The listing builds one solid part. Answer for the finished solid, in the listing's coordinates (mm). A direction names the side the tool comes from. Give positions to 0.01 mm unless a question says otherwise; leave off trailing zeros. Order: outer loops, then holes, each group sorted by start corner. A loop starts at its lowest first (then second) coordinate and runs counter-clockwise, first axis right, second up.
```python
from build123d import *

# Parameters (mm, degrees)
F1_DEPTH = 12.7
F3_DEPTH = 25.4
F4_R     = 4.8895
F5_DEPTH = 25.4


with BuildPart() as f1:
    # F0 (on Top) → F1 (new body)
    with BuildSketch(Plane.XY):
        Polygon((222.6329271213, 5.3004485337), (222.6329271213, 0), (222.6329271213, -5.3004485337), (222.6329271213, -30.3229389596), (285.3670728787, -30.3229389596), (285.3670728787, 30.3229389596), (222.6329271213, 30.3229389596), align=None)
        with BuildLine():
            ThreePointArc((44.1328420266, 5.3004485337), (44.3706396623, 2.654964399), (44.45, 0))
            Line((44.45, 0), (222.6329271213, 0))
            Line((222.6329271213, 0), (222.6329271213, 5.3004485337))
            Line((222.6329271213, 5.3004485337), (44.1328420266, 5.3004485337))
        make_face()
        with BuildLine():
            Line((222.6329271213, 0), (44.45, 0))
            ThreePointArc((44.45, 0), (44.3706396623, -2.654964399), (44.1328420266, -5.3004485337))
            Line((44.1328420266, -5.3004485337), (222.6329271213, -5.3004485337))
            Line((222.6329271213, -5.3004485337), (222.6329271213, 0))
        make_face()
        with BuildLine():
            ThreePointArc((-38.8833935549, 5.3004485337), (0, 39.243), (38.8833935548, 5.3004485337))
            Line((38.8833935548, 5.3004485337), (44.1328420266, 5.3004485337))
            ThreePointArc((44.1328420266, 5.3004485337), (0, 44.45), (-44.1328420266, 5.3004485337))
            Line((-44.1328420266, 5.3004485337), (-38.8833935549, 5.3004485337))
        make_face()
        with BuildLine():
            Line((44.1328420266, -5.3004485337), (38.8833935548, -5.3004485337))
            ThreePointArc((38.8833935548, -5.3004485337), (0, -39.243), (-38.8833935549, -5.3004485337))
            Line((-38.8833935549, -5.3004485337), (-44.1328420266, -5.3004485337))
            ThreePointArc((-44.1328420266, -5.3004485337), (0, -44.45), (44.1328420266, -5.3004485337))
        make_face()
        with BuildLine():
            ThreePointArc((38.8833935548, 5.3004485337), (39.1529951745, 2.656316597), (39.243, 0))
            Line((39.243, 0), (44.45, 0))
            ThreePointArc((44.45, 0), (44.3706396623, 2.654964399), (44.1328420266, 5.3004485337))
            Line((44.1328420266, 5.3004485337), (38.8833935548, 5.3004485337))
        make_face()
        with BuildLine():
            Line((44.45, 0), (39.243, 0))
            ThreePointArc((39.243, 0), (39.1529951745, -2.656316597), (38.8833935548, -5.3004485337))
            Line((38.8833935548, -5.3004485337), (44.1328420266, -5.3004485337))
            ThreePointArc((44.1328420266, -5.3004485337), (44.3706396623, -2.654964399), (44.45, 0))
        make_face()
        with BuildLine():
            ThreePointArc((-38.8833935549, -5.3004485337), (-39.243, 0), (-38.8833935549, 5.3004485337))
            Line((-38.8833935549, 5.3004485337), (-44.1328420266, 5.3004485337))
            ThreePointArc((-44.1328420266, 5.3004485337), (-44.45, 0), (-44.1328420266, -5.3004485337))
            Line((-44.1328420266, -5.3004485337), (-38.8833935549, -5.3004485337))
        make_face()
    extrude(amount=F1_DEPTH)

    # F2 (on face) → F3 (cut)
    with BuildSketch(Plane.XY.offset(12.7)):
        with BuildLine():
            ThreePointArc((261.2282336072, -15.141530461), (269.1570726001, -9.3443922439), (272.182900235, 0))
            ThreePointArc((272.182900235, 0), (269.1570726001, 9.3443922439), (261.2282336072, 15.141530461))
            Line((261.2282336072, 15.141530461), (261.2282336072, -15.141530461))
        make_face()
    extrude(amount=-F3_DEPTH, mode=Mode.SUBTRACT)

    # F4 (on face) → F5 (cut)
    with BuildSketch(Plane.YZ.offset(285.3670728787)):
        with Locations((0, 6.35)):
            Circle(F4_R)
    extrude(amount=-F5_DEPTH, mode=Mode.SUBTRACT)


solid = f1.part
```
1) Straight lines are drawn through the part: probe 1 along Z at (x, y) = (281, 0); probe 2 along X at (y, z) = (8, 9.75); probe 3 along X at (y, z) = (25, 8.5). For each, find the intervals that lie inside material, in ascending order.
Geometry says:
probe 1: z = 0 to 1.46, 11.24 to 12.7
probe 2: x = -43.72 to -38.42, 38.42 to 43.72, 222.63 to 261.23, 270.03 to 285.37
probe 3: x = -36.75 to -30.25, 30.25 to 36.75, 222.63 to 285.37
2) Find section C-C (x = 167.5). Write down the section's boundary in (y, z), then the cut area to 3 significant figures.
Geometry says:
outline: (-5.3, 0) - (5.3, 0) - (5.3, 12.7) - (-5.3, 12.7) - close
area: 135 mm2
3) Find section B-B (y = -27.5). Write down the section's boundary in (x, z).
Geometry says:
outline: (-34.92, 0) - (-28, 0) - (-28, 12.7) - (-34.92, 12.7) - close; (28, 0) - (34.92, 0) - (34.92, 12.7) - (28, 12.7) - close; (222.63, 0) - (285.37, 0) - (285.37, 12.7) - (222.63, 12.7) - close
4) For a pull along Z with two mould halves and no side action, classify faces 6 (the cylindrical face through (278.488, -0.637, 11.198)), 7 (the flat face through (169, 0, 12.7)), 8 (the flat face through (169, 0, 0)), 9 (the flat face through (285.367, 0, 12)) as +Z half, -Z half, draft (parallel to the pull), parting line (faces both ways), or undercut.
Geometry says:
face 6: undercut
face 7: +Z half
face 8: -Z half
face 9: draft
5) A tool of negligible diameter and unlimited length cuts with its end or side. For faces 1 (the flat face through (261.228, 4, 11)), 2 (the flat face through (135, 5.3, 6)), 3 (the flat face through (132, -5.3, 6)), 4 (the flat face through (254, 30.323, 6)), 5 (the flat face through (259.967, 0, 6)), from which of +Z, -Z, +X, -X, +Y, -Y can it reach the whole face along a straight path? Write none if from no direction.
Geometry says:
face 1: +Z, -Z
face 2: +Z, -Z, +Y
face 3: +Z, -Z, -Y
face 4: +Z, -Z, +X, +Y
face 5: +X
6) Given P1, Ø1, axis at x = 153, z = 5.5, coming from the +Y side; P2, Ø4, axis at x = 250, z = 8, coming from the +Y side; P3, Ø6.5, axis at y = -23.5, z = 8.5, coming from the -X side, each flat-ended and moving along its own axis, determine where each tip first touches the part or whether it passes through.
Geometry says:
P1: stops at y = 5.3
P2: stops at y = 30.32
P3: stops at x = -39.57
7) Find section A-A (z = 6.35). Write down the section's boundary in (x, y).
Geometry says:
outline: (44.13, -5.3) - (222.63, -5.3) - (222.63, -30.32) - (285.37, -30.32) - (285.37, -4.89) - (271.41, -4.89) arc R15.94 cw to (261.23, -15.14) - (261.23, -4.89) - (259.97, -4.89) - (259.97, 4.89) - (261.23, 4.89) - (261.23, 15.14) arc R15.94 cw to (271.41, 4.89) - (285.37, 4.89) - (285.37, 30.32) - (222.63, 30.32) - (222.63, 5.3) - (44.13, 5.3) arc R44.45 ccw (long way) to start; hole circle Ø78.49 at (0, 0)
